```python
from build123d import *

# Parameters (mm, degrees)
CROQUIS1_R              = 7.5
EXTRUIR1_DEPTH          = 10
EXTRUIR2_DEPTH          = 10
CROQUIS3_R              = 30
EXTRUIR3_DEPTH          = 9
REDONDEO1_R             = 5
EXTRUIR4_DEPTH          = 10
REDONDEO2_R             = 2
CROQUIS5_R              = 39.877660951
CORTAR_EXTRUIR1_DEPTH   = 10
CROQUIS7_W              = 10
CROQUIS7_H              = 50
SALIENTE_EXTRUIR1_DEPTH = 2
CROQUIS8_W              = 50
CROQUIS8_H              = 10
SALIENTE_EXTRUIR2_DEPTH = 2
CROQUIS10_R             = 1.55
CORTAR_EXTRUIR2_DEPTH   = 2


with BuildPart() as part:
    # Croquis1 → Extruir1 (new body)
    with BuildSketch(Plane(origin=(0, 0, 0), x_dir=(1, 0, 0), z_dir=(0, 1, 0))):
        Circle(CROQUIS1_R)
    extrude(amount=EXTRUIR1_DEPTH)

    # Croquis2 → Extruir2 (cut)
    with BuildSketch(Plane(origin=(0, 10, 0), x_dir=(1, 0, 0), z_dir=(0, 1, 0))):
        with BuildLine():
            Line((-1.9, 2.05669638), (-1.9, -2.05669638))
            ThreePointArc((-1.9, -2.05669638), (0, -2.8), (1.9, -2.05669638))
            Line((1.9, -2.05669638), (1.9, 2.05669638))
            ThreePointArc((1.9, 2.05669638), (0, 2.8), (-1.9, 2.05669638))
        make_face()
    extrude(amount=-EXTRUIR2_DEPTH, mode=Mode.SUBTRACT)

    # Croquis3 → Extruir3 (add)
    with BuildSketch(Plane.XZ):
        Circle(CROQUIS3_R)
    extrude(amount=EXTRUIR3_DEPTH)

    # Redondeo1
    redondeo1_edges = [part.edges().sort_by_distance(p)[0] for p in [
        (-7.5, 0, 0),
    ]]
    fillet(redondeo1_edges, radius=REDONDEO1_R)

    # Croquis4 → Extruir4 (cut)
    with BuildSketch(Plane(origin=(0, 0, 0), x_dir=(1, 0, 0), z_dir=(0, 1, 0))):
        with BuildLine():
            ThreePointArc((-13.896428557, -5.647058824), (-10.606601718, -10.606601718), (-5.647058824, -13.896428557))
            ThreePointArc((-5.647058824, -13.896428557), (-2.209821435, -22.039548299), (-10.352941176, -25.476785688))
            ThreePointArc((-10.352941176, -25.476785688), (-19.445436483, -19.445436483), (-25.476785688, -10.352941176))
            ThreePointArc((-25.476785688, -10.352941176), (-22.039548299, -2.209821435), (-13.896428557, -5.647058824))
        make_face()
        with BuildLine():
            ThreePointArc((-5.647058824, 13.896428557), (-2.209821435, 22.039548299), (-10.352941176, 25.476785688))
            ThreePointArc((-10.352941176, 25.476785688), (-19.445436483, 19.445436483), (-25.476785688, 10.352941176))
            ThreePointArc((-25.476785688, 10.352941176), (-22.039548299, 2.209821435), (-13.896428557, 5.647058824))
            ThreePointArc((-13.896428557, 5.647058824), (-10.606601718, 10.606601718), (-5.647058824, 13.896428557))
        make_face()
        with BuildLine():
            ThreePointArc((10.352941176, 25.476785688), (2.209821435, 22.039548299), (5.647058824, 13.896428557))
            ThreePointArc((5.647058824, 13.896428557), (10.606601718, 10.606601718), (13.896428557, 5.647058824))
            ThreePointArc((13.896428557, 5.647058824), (22.039548299, 2.209821435), (25.476785688, 10.352941176))
            ThreePointArc((25.476785688, 10.352941176), (19.445436483, 19.445436483), (10.352941176, 25.476785688))
        make_face()
        with BuildLine():
            ThreePointArc((5.647058824, -13.896428557), (2.209821435, -22.039548299), (10.352941176, -25.476785688))
            ThreePointArc((10.352941176, -25.476785688), (19.445436483, -19.445436483), (25.476785688, -10.352941176))
            ThreePointArc((25.476785688, -10.352941176), (22.039548299, -2.209821435), (13.896428557, -5.647058824))
            ThreePointArc((13.896428557, -5.647058824), (10.606601718, -10.606601718), (5.647058824, -13.896428557))
        make_face()
    extrude(amount=-EXTRUIR4_DEPTH, mode=Mode.SUBTRACT)

    # Redondeo2
    redondeo2_edges = [part.edges().sort_by_distance(p)[0] for p in [
        (-30, 0, 0),
        (-30, -9, 0),
    ]]
    fillet(redondeo2_edges, radius=REDONDEO2_R)

    # Croquis5 → Cortar-Extruir1 (cut)
    with BuildSketch(Plane.XZ.offset(9)):
        Circle(CROQUIS5_R)
    extrude(amount=-CORTAR_EXTRUIR1_DEPTH, mode=Mode.SUBTRACT)

    # Croquis7 → Saliente-Extruir1 (add)
    with BuildSketch(Plane.XZ.offset(-1)):
        Rectangle(CROQUIS7_W, CROQUIS7_H)
    extrude(amount=-SALIENTE_EXTRUIR1_DEPTH)

    # Croquis8 → Saliente-Extruir2 (add)
    with BuildSketch(Plane.XZ.offset(-1)):
        Rectangle(CROQUIS8_W, CROQUIS8_H)
    extrude(amount=-SALIENTE_EXTRUIR2_DEPTH)

    # Croquis10 → Cortar-Extruir2 (cut)
    with BuildSketch(Plane.XZ.offset(-1)):
        with Locations((-18, 0)):
            Circle(CROQUIS10_R)
        with Locations((0, 18)):
            Circle(CROQUIS10_R)
        with Locations((0, -18)):
            Circle(CROQUIS10_R)
        with Locations((18, 0)):
            Circle(CROQUIS10_R)
    extrude(amount=-CORTAR_EXTRUIR2_DEPTH, mode=Mode.SUBTRACT)


solid = part.part
```
Can you work these out from the model? Positions are in its coordinate system, mm. A direction names the side the tool comes from. Give positions to 0.01 mm unless a question says otherwise; leave off trailing zeros. Write each loop counter-clockwise with the first axis right and the second up, starting at its lowest first coordinate (ties: lowest second). Pieces come first, ordered by that corner, then holes. Notation, with made-up numbers: (17.25, 29) -> (41.25, 29) arc R22 ccw to (41.25, 61) -> close; hole circle Ø3 at (-3, -23). An arc over 180 degrees is marked (long way). Write item = value, one per line.
(1) Suppose I cut it at C-C on y = 7. Write out the boundary of the cut face in (x, z), then the cut area to 3 significant figures.
Worked out:
outline = circle Ø15 at (0, 0); hole (-1.9, -2.06) arc R2.8 ccw to (1.9, -2.06) -> (1.9, 2.06) arc R2.8 ccw to (-1.9, 2.06) -> close
area = 157 mm^2
(2) Thinking about a two-plate mould opening in Z: for faces 1 (the face through (3, 10, 0)), 2 (the face through (-16, 2, -5)), 3 (the face through (-7.493, 7.465, -0.33)), 4 (the face through (1.9, 7, 0)), which applies, released by +Z, released by -Z, zero draft, split by the parting line, or undercut?
Worked out:
face_1 = zero draft
face_2 = released by -Z
face_3 = split by the parting line
face_4 = undercut
(3) I'm going to push flat-ended pins straight in: P1, Ø3, axis at x = -5, z = -18, coming from the +Y side; P2, Ø1, axis at y = 2, z = -12, coming from the +X side; P3, Ø1.2, axis at y = 8, z = -0.5, coming from the +X side; P4, Ø5, axis at x = 11.5, y = 6, coming from the -Z side. Where does each tip first touch, or does it pass through?
Worked out:
P1 = 3
P2 = 5
P3 = 7.5
P4 = through
(4) Suppose I cut it at A-A on x = -18. Write out the boundary of the cut face in (y, z), then the cut area to 3 significant figures.
Worked out:
outline = (1, -5) -> (3, -5) -> (3, -1.55) -> (1, -1.55) -> close; (1, 1.55) -> (3, 1.55) -> (3, 5) -> (1, 5) -> close
area = 13.8 mm^2
(5) For faces 5 (the face through (-1.9, 7, 0)), 6 (the face through (-0.202, 1.986, -16.463)), which set-ups out of +Z, -Z, +X, -X, +Y, -Y let a thin tool reach every point of the face, with its end or its side?
Worked out:
face_5 = +Y
face_6 = +Y, -Y
(6) I need wall thicknesses on probe 1 along Z at (x, y) = (0, 1.85); probe 2 along Z at (x, y) = (1.5, 5.5); probe 3 along Y at (x, z) = (-20, -2.5). Which ranges of each line are inside material? Lowest first, please. Write a range as from..to.
Worked out:
probe_1 = -25..-19.55, -16.45..16.45, 19.55..25
probe_2 = -7.35..-2.36, 2.36..7.35
probe_3 = 1..3
(7) Suppose I cut it at D-D on x = 0. Write out the boundary of the cut face in (y, z), then the cut area to 3 significant figures.
Worked out:
outline = (1, -25) -> (3, -25) -> (3, -19.55) -> (1, -19.55) -> close; (1, -16.45) -> (3, -16.45) -> (3, -7.92) arc R5 cw to (5, -7.5) -> (10, -7.5) -> (10, -2.8) -> (3, -2.8) -> (3, 2.8) -> (10, 2.8) -> (10, 7.5) -> (5, 7.5) arc R5 cw to (3, 7.92) -> (3, 16.45) -> (1, 16.45) -> close; (1, 19.55) -> (3, 19.55) -> (3, 25) -> (1, 25) -> close
area = 154 mm^2
(8) Suppose I cut it at B-B on z = -18. Write out the boundary of the cut face in (x, y).
Worked out:
outline = (-5, 1) -> (-1.55, 1) -> (-1.55, 3) -> (-5, 3) -> close; (1.55, 1) -> (5, 1) -> (5, 3) -> (1.55, 3) -> close
